Autodesk Inventor part; units mm, degrees
ref_plane "YZ Plane" through (0, 0, 0) normal (1, 0, 0) x (0, 1, 0)
ref_plane "XZ Plane" through (0, 0, 0) normal (0, 1, 0) x (-1, 0, 0)
ref_plane "XY Plane" through (0, 0, 0) normal (0, 0, 1) x (1, 0, 0)
sketch "スケッチ1" plane through (0, 0, 0) normal (0, 0, 1) x (1, 0, 0)
  circle A0 centre (0, 0) radius 10
  circle A1 centre (0, 0) radius 13 construction
  line L0 (0, 0) -> (0, -7.3396) construction
  circle A2 centre (9.1924, -9.1924) radius 1.55 construction
  line L1 (0, 0) -> (9.1924, -9.1924) construction
  circle A3 centre (9.1924, 9.1924) radius 1.55 construction
  circle A4 centre (-9.1924, 9.1924) radius 1.55 construction
  circle A5 centre (-9.1924, -9.1924) radius 1.55 construction
  line L2 (-24.5, 0) -> (24.5, 0)
  circle A6 centre (0, 22.5) radius 4
  circle A7 centre (0, -22.5) radius 4
  circle A8 centre (0, 0) radius 16 construction
  circle A9 centre (0, 0) radius 17.5
  line L3 (-3.2, 24.9) -> (-14, 10.5)
  line L4 (-3.2, -24.9) -> (-14, -10.5)
  line L5 (3.2, -24.9) -> (14, -10.5)
  line L6 (3.2, 24.9) -> (14, 10.5)
  dimension "d3" = 26
  dimension "d2" = 20
  dimension "d4" = 3.1
  dimension "d5" = 45
  dimension "d9" = 360
  dimension "d13" = 45
  dimension "d14" = 8
  dimension "d15" = 8
  dimension "d16" = 32
  dimension "d17" = 35
extrude "押し出し1" add sketch "スケッチ1" along normal blind 2 contours L2 A9 A0 | A0 L2 A9 | A9 L3 A6 L6 | L5 A7 L4 A9 | A6 | A7
hole "穴1" at (9.1924, -9.1924, 0) at (-9.1924, -9.1924, 0) at (9.1924, 9.1924, 0) at (-9.1924, 9.1924, 0) at (0, 22.5, 0) at (0, -22.5, 0) direction (0, 0, 1) diameter 3.05 end through all
properties part number "al_motorbase_1" material "アルミニウム 6061-AHC"
Model file for the job. Use its own axes, mm. Round coordinates to 2 decimals unless told otherwise and drop trailing zeros. Order: outer loops, then holes, each group sorted by start corner. A loop starts at its lowest first (then second) coordinate and runs counter-clockwise, first axis right, second up. Notation, with made-up numbers: M -23.5,44 L 3.5,44 A16 ccw 3.5,60 Z; hole C 46.5,87.5 d6. An arc over 180 degrees is marked long. Write each question's results on one line, items separated by ' | '. Start each with the question number.
(1) Saw through at B-B, the plane x = 0. Give the cut face in (y, z) (3 decimals).
(2) Saw through at A-A, the plane y = -22.5. Give the cut face in (x, z) (3 decimals), then the cut area to 3 significant figures.
(3) Saw through at C-C, the plane z = 0.4. Give the cut face in (x, y) (3 decimals), then the cut area to 3 significant figures.
(4) Saw through at D-D, the plane y = 23.5. Give the cut face in (x, z).
(5) Two-plate mould, pull along Y, no slides. Class faces 1 (the face through (-17.5, -0.2, 1)), 2 (the face through (-8.524, 17.801, 0.986)), 3 (the face through (-2.17, 9.76, 0.99)): pulls with the +Y half, pulls with the -Y half, needs draft (parallel to the pull), parting line crosses it, or undercut.
(6) Probe probe 1 along Y at (x, z) = (8.5, 0.85); probe 2 along X at (y, z) = (-8.5, 0.5); probe 3 along Y at (x, z) = (0.5, 1). List the from-to ranges inside material, lowest first. Write a range as from..to.
Established:
1) outline: M -26.5,0 L -24.025,0 L -24.025,2 L -26.5,2 Z; M -20.975,0 L -10,0 L -10,2 L -20.975,2 Z; M 10,0 L 20.975,0 L 20.975,2 L 10,2 Z; M 24.025,0 L 26.5,0 L 26.5,2 L 24.025,2 Z
2) outline: M -5,0 L -1.525,0 L -1.525,2 L -5,2 Z; M 1.525,0 L 5,0 L 5,2 L 1.525,2 Z | area: 13.9 mm^2
3) outline: M -14,-10.5 L -3.2,-24.9 A4 ccw 3.2,-24.9 L 14,-10.5 A17.5 ccw 14,10.5 L 3.2,24.9 A4 ccw -3.2,24.9 L -14,10.5 A17.5 ccw Z; hole C -9.192,-9.192 d3.05; hole C -9.192,9.192 d3.05; hole C 0,0 d20; hole C 0,-22.5 d3.05; hole C 0,22.5 d3.05; hole C 9.192,-9.192 d3.05; hole C 9.192,9.192 d3.05 | area: 840 mm^2
4) outline: M -4.25,0 L -1.15,0 L -1.15,2 L -4.25,2 Z; M 1.15,0 L 4.25,0 L 4.25,2 L 1.15,2 Z
5) face 1: parting line crosses it | face 2: pulls with the +Y half | face 3: undercut
6) probe 1: y = -17.83..-10.55, -7.83..-5.27, 5.27..7.83, 10.55..17.83 | probe 2: x = -15.3..-10.55, -7.83..-5.27, 5.27..7.83, 10.55..15.3 | probe 3: y = -26.47..-23.94, -21.06..-9.99, 9.99..21.06, 23.94..26.47
